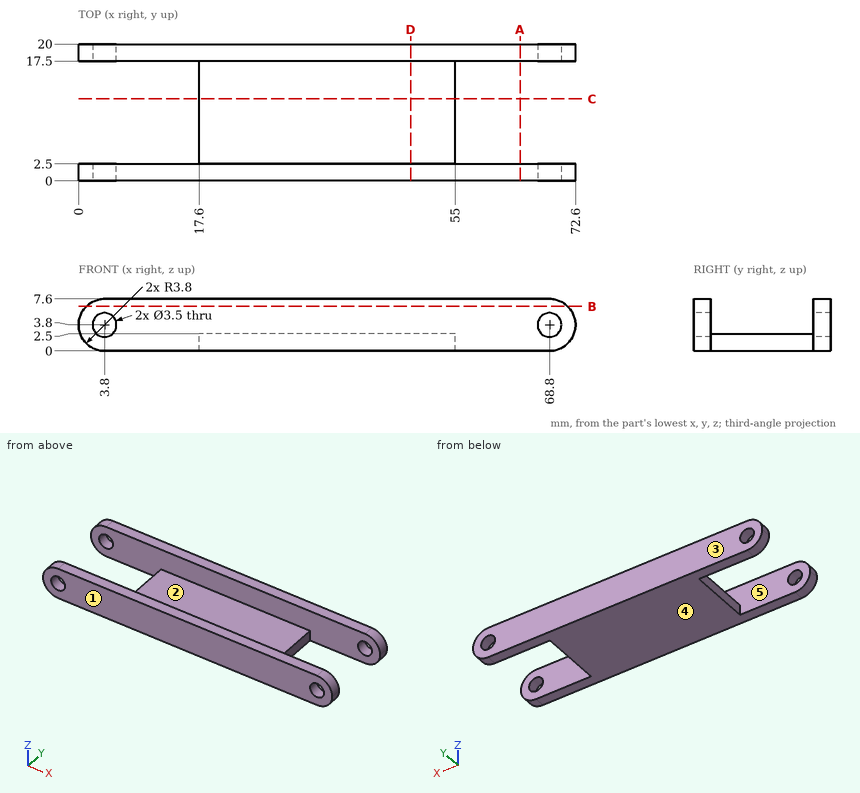
Could you check a few things on this drawing? It's one solid part, dimensions in mm from its lowest x, y, z. A direction names the side the tool comes from. Round coordinates to 2 decimals unless told otherwise and drop trailing zeros. Loops run counter-clockwise (first coordinate to the right, second up) from the corner with the lowest first, then second, coordinate; pieces in that order, holes last. Notation, with made-up numbers: (10, 86.5) -> (42, 86.5) arc R11 ccw to (42, 94.5) -> close; hole circle Ø11 at (37.25, 84). An arc over 180 degrees is marked (long way). One line per item, written item: value. Start each with the question number.
1. If we section it at B-B, the plane z = 6.5: Write out the boundary of the cut face in (x, y), then the cut area to 3 significant figures.
2. If I drill on probe 1 along Y at (x, z) = (26, 5.25); probe 2 along X at (y, z) = (19.25, 3.5); probe 3 along Z at (x, y) = (20, 10.75), over which ranges is the centre line in solid material (lowest first)?
3. If we section it at A-A, the plane x = 64.5: Write out the boundary of the cut face in (y, z).
4. If we mould it in two halves opening along Y, with no side actions, what happens to the marked faces 3, 4 and 5? For each: pulls with the +Y half, pulls with the -Y half, needs draft (parallel to the pull), parting line crosses it, or undercut.
5. For the marked faces 1 and 2, which set-ups out of +Z, -Z, +X, -X, +Y, -Y let a thin tool reach every point of the face, with its end or its side?
6. If we section it at D-D, the plane x = 48.5: Write out the boundary of the cut face in (y, z).
7. For pin 1 (1.5 mm diameter, centred on x = 23, z = 2.5, fed in from -Y); pin 2 (6 mm diameter, centred on x = 23, y = 11.5, fed in from +Z); pin 3 (2 mm diameter, centred on y = 6.5, z = 0.5, fed in from +X); pin 4 (3 mm diameter, centred on y = 8, z = 3, fed in from -X), each with a flat end and sliding along its axis, tell me the tip position at first contact or that it passes through.
8. If we section it at C-C, the plane y = 12: Write out the boundary of the cut face in (x, z).
Calculated:
1. outline: (1.13, 0) -> (71.47, 0) -> (71.47, 2.5) -> (1.13, 2.5) -> close; (1.13, 17.5) -> (71.47, 17.5) -> (71.47, 20) -> (1.13, 20) -> close
1. area: 352 mm²
2. probe 1: y = 0 to 2.5, 17.5 to 20
2. probe 2: x = 0.01 to 2.08, 5.52 to 67.08, 70.52 to 72.59
2. probe 3: z = 0 to 2.5
3. outline: (0, 0) -> (2.5, 0) -> (2.5, 7.6) -> (0, 7.6) -> close; (17.5, 0) -> (20, 0) -> (20, 7.6) -> (17.5, 7.6) -> close
4. face 3: pulls with the +Y half
4. face 4: needs draft
4. face 5: undercut
5. face 1: +Z, -Z, +X, -X, -Y
5. face 2: +Z, +X, -X
6. outline: (0, 0) -> (20, 0) -> (20, 7.6) -> (17.5, 7.6) -> (17.5, 2.5) -> (2.5, 2.5) -> (2.5, 7.6) -> (0, 7.6) -> close
7. pin 1: stops at y = 0
7. pin 2: stops at z = 2.5
7. pin 3: stops at x = 55
7. pin 4: stops at x = 17.6
8. outline: (17.6, 0) -> (55, 0) -> (55, 2.5) -> (17.6, 2.5) -> close
